```python
from build123d import *

# Parameters (mm, degrees)
BOSS_EXTRUDE1_DEPTH = 5
SKETCH2_W           = 5
SKETCH2_H           = 20
SKETCH2_H_2         = 5
SKETCH2_W_2         = 20
BOSS_EXTRUDE2_DEPTH = 44
SKETCH3_R           = 2
CUT_EXTRUDE1_DEPTH  = 53.306787322
FILLET1_R           = 3
FILLET2_R           = 3


with BuildPart() as part:
    # Sketch1 → Boss-Extrude1 (new body)
    with BuildSketch(Plane(origin=(0, 0, 0), x_dir=(1, 0, 0), z_dir=(0, 1, 0))):
        Polygon((20, 20), (-20, 20), (-20, -20), (0, -20), (0, 0), (20, 0), align=None)
    extrude(amount=BOSS_EXTRUDE1_DEPTH)

    # Sketch2 → Boss-Extrude2 (add)
    with BuildSketch(Plane(origin=(0, 5, 0), x_dir=(1, 0, 0), z_dir=(0, 1, 0))):
        with Locations((-2.5, -10)):
            Rectangle(SKETCH2_W, SKETCH2_H)
        with Locations((-2.5, 2.5)):
            Rectangle(SKETCH2_W, SKETCH2_H_2)
        with Locations((10, 2.5)):
            Rectangle(SKETCH2_W_2, SKETCH2_H_2)
    extrude(amount=BOSS_EXTRUDE2_DEPTH)

    # Sketch3 → Cut-Extrude1 (cut, through all)
    with BuildSketch(Plane(origin=(0, 5, 0), x_dir=(1, 0, 0), z_dir=(0, 1, 0))):
        with Locations(Location((-12.5, -12, 0), (0, 0, 270))):
            Circle(SKETCH3_R)
        with Locations(Location((-12.5, 12.5, 0), (0, 0, 270))):
            Circle(SKETCH3_R)
        with Locations(Location((12, 12.5, 0), (0, 0, 270))):
            Circle(SKETCH3_R)
        with Locations(Location((-12.5, 0, 0), (0, 0, 270))):
            Circle(SKETCH3_R)
        with Locations(Location((0, 12.5, 0), (0, 0, 270))):
            Circle(SKETCH3_R)
    extrude(amount=-CUT_EXTRUDE1_DEPTH, mode=Mode.SUBTRACT)

    # Fillet1
    fillet1_edges = [part.edges().sort_by_distance(p)[0] for p in [
        (7.5, 5, -5),
        (-5, 5, 7.5),
    ]]
    fillet(fillet1_edges, radius=FILLET1_R)

    # Fillet2
    fillet2_edges = [part.edges().sort_by_distance(p)[0] for p in [
        (-20, 2.5, -20),
    ]]
    fillet(fillet2_edges, radius=FILLET2_R)


solid = part.part
```
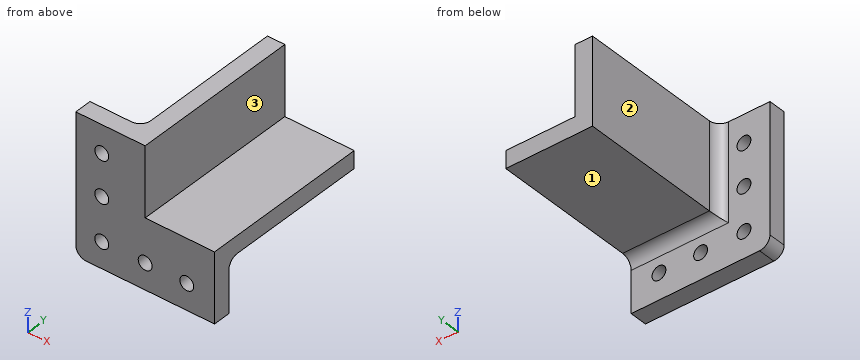
Can you work these out from the model? Positions are in its coordinate system, mm. Face numbers are marked on the shaded views. A direction names the side the tool comes from. Round coordinates to 2 decimals unless told otherwise and drop trailing zeros. Loops run counter-clockwise (first coordinate to the right, second up) from the corner with the lowest first, then second, coordinate; pieces in that order, holes last. Notation, with made-up numbers: M 37.25,70 L 41.25,70 A19 ccw 41.25,75 Z; hole C -13,-14.5 d8. An arc over 180 degrees is marked long. Answer in a Markdown table with one row per item.
1. Please list where these lines run through material, in increasing order: line 1 (X direction, y = 3, z = -12); line 2 (Y direction, x = 15.5, z = -10); line 3 (Z direction, x = 14, y = 45.5). Write a range as from..to.
Established:
| item | result |
|---|---|
| line 1 | -20..-14.44, -10.56..-1.94, 1.94..10.06, 13.94..20 |
| line 2 | 0..5 |
| line 3 | -5..0 |
2. If we section it at C-C, the plane x = 12: Please give me the cut outline in (y, z).
Established:
| item | result |
|---|---|
| outline | M 0,-20 L 5,-20 L 5,-14.5 L 0,-14.5 Z; M 0,-10.5 L 5,-10.5 L 5,-8 A3 cw 8,-5 L 49,-5 L 49,0 L 0,0 Z |
3. If we section it at A-A, the plane z = -12.5: Please give me the cut outline in (x, y).
Established:
| item | result |
|---|---|
| outline | M -20,0 L -14.5,0 L -14.5,5 L -20,5 Z; M -10.5,0 L -2,0 L -2,5 L -10.5,5 Z; M 2,0 L 10,0 L 10,5 L 2,5 Z; M 14,0 L 20,0 L 20,5 L 14,5 Z |
4. I'm going to push flat-ended pins straight in: pin 1 Ø1.5 at (x, y) = (15.5, 12) entering from +Z; pin 2 Ø10 at (y, z) = (42.5, 6.5) entering from -X; pin 3 Ø12.5 at (x, y) = (7.5, 38) entering from -Z. Where does each tip first touch, or does it pass through?
Established:
| item | result |
|---|---|
| pin 1 | z = 0 |
| pin 2 | x = -5 |
| pin 3 | z = -5 |
5. If we section it at D-D, the plane z = 12: Please give me the cut outline in (x, y), plus the area to 3 significant figures.
Established:
| item | result |
|---|---|
| outline | M -20,0 L -14.5,0 L -14.5,5 L -20,5 Z; M -10.5,0 L 0,0 L 0,49 L -5,49 L -5,8 A3 cw -8,5 L -10.5,5 Z |
| area | 302 mm² |
6. On a 3-axis mill with a long thin cutter (end or side, diameter ignored), from which of +Z, -Z, +X, -X, +Y, -Y can I reach the whole of each face in a straight line? I mean the marked faces 1, 2 and 3. Say none if no direction works.
Established:
| item | result |
|---|---|
| face 1 | -Z, +X, -X, +Y |
| face 2 | +Z, -Z, -X, +Y |
| face 3 | +Z, +X, +Y, -Y |
7. If we section it at B-B, the plane x = -12.5: Please give me the cut outline in (y, z), plus the area to 3 significant figures.
Established:
| item | result |
|---|---|
| outline | M 0,-20 L 5,-20 L 5,-14.5 L 0,-14.5 Z; M 0,-10.5 L 5,-10.5 L 5,-2 L 0,-2 Z; M 0,2 L 5,2 L 5,10 L 0,10 Z; M 0,14 L 5,14 L 5,20 L 0,20 Z |
| area | 140 mm² |
